Input: part model. Units: mm. Frame: model coordinates. Round coordinates to 2 decimals unless told otherwise and drop trailing zeros. Order: outer loops, then holes, each group sorted by start corner. A loop starts at its lowest first (then second) coordinate and runs counter-clockwise, first axis right, second up. Notation, with made-up numbers: (-3, 67.25) -> (20, 67.25) arc R23 cw to (20, 92.25) -> close; hole circle Ø1 at (5.25, 79.25). An arc over 180 degrees is marked (long way). Use a Markdown table: item, result.
Autodesk Inventor part; units mm, degrees
ref_plane "YZ Plane" through (0, 0, 0) normal (1, 0, 0) x (0, 1, 0)
ref_plane "XZ Plane" through (0, 0, 0) normal (0, 1, 0) x (-1, 0, 0)
ref_plane "XY Plane" through (0, 0, 0) normal (0, 0, 1) x (1, 0, 0)
sketch "Sketch1" plane through (0, 0, 0) normal (0, 0, 1) x (1, 0, 0)
  circle A0 centre (0, 0) radius 45
  line L0 (0, -45) -> (43, -45)
  line L1 (43, -45) -> (43, -25)
  line L2 (43, -25) -> (0, -25)
  line L3 (0, -25) -> (0, -45)
  line L4 (0, 45) -> (1850, 45)
  line L5 (1850, 45) -> (1850, 25)
  line L6 (1850, 25) -> (0, 25)
  line L7 (0, 25) -> (0, 45)
  circle A1 centre (0, 0) radius 25
  point P0 (0, -25)
  point P1 (0, 25)
  point P2 (13, -25)
  point P3 (-45, 0)
  dimension "d0" = 90
  dimension "d1" = 20
  dimension "d2" = 20
  dimension "d9" = 1850
  dimension "d10" = 58
  dimension "d11" = 30
extrude "Extrusion1" add sketch "Sketch1" along normal blind 39 contours L7 A1 L3 A0 | L4 L5 L6 A0 | A0 L6 L7 | L3 L2 A0 | A0 L2 L1 L0
properties part number "J15BF.1.30_Yaxis"
1) Cut plane C-C on y = 0. Return loops of the section in (x, z), and give its area (3 significant figures).
Results found:
| item | result |
|---|---|
| outline | (-45, 0) -> (-25, 0) -> (-25, 39) -> (-45, 39) -> close |
| area | 780 mm² |
2) Pull-direction query (Y, two-part tool) for faces 1 (the flat face through (912, 45, 19)), 2 (the flat face through (828, 34, 39)), 3 (the flat face through (22, -25, 19)); classes: +Y half, -Y half, draft (parallel to the pull), parting line (faces both ways), or undercut.
Results found:
| item | result |
|---|---|
| face 1 | +Y half |
| face 2 | draft |
| face 3 | undercut |
3) Pin query (flat end, axial travel): pin 1 Ø1 at (y, z) = (16, 10.5) entering from +X; pin 2 Ø6 at (y, z) = (-32, 26) entering from +X; pin 3 Ø1 at (y, z) = (9, 8) entering from +X. Return the tip coordinate at first contact, or that it passes through.
Results found:
| item | result |
|---|---|
| pin 1 | stops at x = -18.78 |
| pin 2 | stops at x = 43 |
| pin 3 | stops at x = -23.12 |
4) Cut plane B-B on x = 1167. Return loops of the section in (y, z).
Results found:
| item | result |
|---|---|
| outline | (25, 0) -> (45, 0) -> (45, 39) -> (25, 39) -> close |
5) Line query: L1, parallel to Y at x = 1599.5, z = 31; L2, parallel to X at y = -17, z = 8; L3, parallel to X at y = -14.5, z = 35. Output: solid intervals per line, ascending. Write a range as [from, to].
Results found:
| item | result |
|---|---|
| L1 | y = [25, 45] |
| L2 | x = [-41.67, -18.33] |
| L3 | x = [-42.6, -20.37] |
6) Cut plane A-A on z = 26.5. Return loops of the section in (x, y), and give its area (3 significant figures).
Results found:
| item | result |
|---|---|
| outline | (0, -45) -> (43, -45) -> (43, -25) -> (0, -25) arc R25 cw to (0, 25) -> (1850, 25) -> (1850, 45) -> (0, 45) arc R45 ccw to start |
| area | 40,100 mm² |
